Source: CAD feature listing. Evaluate the final solid. Frame: model axes, mm. Round coordinates to 2 decimals unless told otherwise and drop trailing zeros. Loops run counter-clockwise (first coordinate to the right, second up) from the corner with the lowest first, then second, coordinate; pieces in that order, holes last. Notation, with made-up numbers: (35, -14) - (40, -14) arc R6 ccw to (40, -7) - close; hole circle Ø5 at (70, 70.5). An arc over 180 degrees is marked (long way). Write item = value, one per line. Start each with the question number.
from build123d import *

# Parameters (mm, degrees)
BOSS_EXTRUDE1_DEPTH = 1.016
FILLET1_R           = 0.635


with BuildPart() as part:
    # Sketch1 → Boss-Extrude1 (new body)
    with BuildSketch(Plane(origin=(0, 0, 0), x_dir=(1, 0, 0), z_dir=(0, 1, 0))):
        with BuildLine():
            Line((0, 0), (-36.068, 0))
            Line((-36.068, 0), (-36.068, 4.826))
            Line((-36.068, 4.826), (-79.248, 4.826))
            Line((-79.248, 4.826), (-79.248, 7.62))
            Line((-79.248, 7.62), (-31.75, 7.62))
            Line((-31.75, 7.62), (-31.75, 3.937))
            ThreePointArc((-31.75, 3.937), (-30.353, 2.54), (-28.956, 3.937))
            Line((-28.956, 3.937), (-28.956, 7.62))
            Line((-28.956, 7.62), (0, 7.62))
            Line((0, 7.62), (0, 0))
        make_face()
    extrude(amount=BOSS_EXTRUDE1_DEPTH)

    # Fillet1
    fillet1_edges = [part.edges().sort_by_distance(p)[0] for p in [
        (0, 0.508, 0),
        (-79.248, 0.508, -4.826),
        (-79.248, 0.508, -7.62),
        (-31.75, 0.508, -7.62),
        (-28.956, 0.508, -7.62),
        (0, 0.508, -7.62),
    ]]
    fillet(fillet1_edges, radius=FILLET1_R)


solid = part.part
(1) Cut plane D-D (x = -31). Output: boundary loops of the cut face in (y, z), and give its area (3 significant figures).
(2) Cut plane A-A (z = -6.25). Output: boundary loops of the cut face in (x, y).
(3) Cut plane C-C (x = -41). Output: boundary loops of the cut face in (y, z), and give its area (3 significant figures).
(4) Mould query, pull axis X, two halves, no side actions, for faces 1 (the face through (-30, 0, -2)), 2 (the face through (-30.38, 0.5, -2.54)). Classes: +X half, -X half, draft (parallel to the pull), parting line (faces both ways), or undercut.
(5) Cut plane B-B (y = 0.2). Output: boundary loops of the cut face in (x, z) (3 decimals).
(6) Material intervals for line 1 along X through (y, z) = (0.35, -5.5); line 2 along X through (y, z) = (0.1, -4.5); line 3 along Z through (x, y) = (-62.5, 0.85), sorted ascending. Write a range as from..to.
Solution:
q1.outline = (0, -2.7) - (1.02, -2.7) - (1.02, 0) - (0, 0) - close
q1.area = 2.74 mm^2
q2.outline = (-79.25, 0) - (-31.75, 0) - (-31.75, 1.02) - (-79.25, 1.02) - close; (-28.96, 0) - (0, 0) - (0, 1.02) - (-28.96, 1.02) - close
q3.outline = (0, -7.62) - (1.02, -7.62) - (1.02, -4.83) - (0, -4.83) - close
q3.area = 2.84 mm^2
q4.face_1 = draft
q4.face_2 = undercut
q5.outline = (-79.248, -6.985) arc R0.635 ccw to (-78.613, -7.62) - (-32.385, -7.62) arc R0.635 ccw to (-31.75, -6.985) - (-31.75, -3.937) arc R1.397 cw to (-28.956, -3.937) - (-28.956, -6.985) arc R0.635 ccw to (-28.321, -7.62) - (-0.635, -7.62) arc R0.635 ccw to (0, -6.985) - (0, -0.635) arc R0.635 ccw to (-0.635, 0) - (-36.068, 0) - (-36.068, -4.826) - (-78.613, -4.826) arc R0.635 ccw to (-79.248, -5.461) - close
q6.line_1 = -79.25..-31.75, -28.96..0
q6.line_2 = -36.07..-31.75, -28.96..0
q6.line_3 = -7.62..-4.83
